```python
from build123d import *

# Parameters (mm, degrees)
EXTRUDE_1_DEPTH     = 12
SKETCH_2_R          = 3
SKETCH_2_R_2        = 0.81
CUT_EXTRUDE_1_DEPTH = 12
CUT_EXTRUDE_2_DEPTH = 8
FILLET_1_R          = 3
SKETCH_4_R          = 2.25
CUT_EXTRUDE_3_DEPTH = 10
CHAMFER_3_SIZE      = 3


with BuildPart() as part:
    # 草图1 → 凸台-拉伸1 (new body)
    with BuildSketch(Plane(origin=(0, 0, 0), x_dir=(1, 0, 0), z_dir=(0, 1, 0))):
        with BuildLine():
            Line((0, 0), (28, 0))
            ThreePointArc((28, 0), (30.121320344, 0.878679656), (31, 3))
            Line((31, 3), (31, 77))
            Line((31, 77), (-3, 77))
            Line((-3, 77), (-3, 3))
            ThreePointArc((-3, 3), (-2.121320344, 0.878679656), (0, 0))
        make_face()
    extrude(amount=EXTRUDE_1_DEPTH)

    # 草图2 → 切除-拉伸1 (cut)
    with BuildSketch(Plane(origin=(14.000000253, 12, -382.2), x_dir=(1, 0, 0), z_dir=(0, 1, 0))):
        with Locations(Location((13, -352.069110398, 0), (0, 0, 270))):
            Circle(SKETCH_2_R)
        with Locations(Location((-13, -352.069110398, 0), (0, 0, 270))):
            Circle(SKETCH_2_R)
        with Locations(Location((13, -378.069110398, 0), (0, 0, 270))):
            Circle(SKETCH_2_R)
        with Locations(Location((-13, -378.069110398, 0), (0, 0, 270))):
            Circle(SKETCH_2_R)
        with Locations(Location((-15.000000143, -309.999984702, 0), (0, 0, 270))):
            Circle(SKETCH_2_R_2)
        with Locations(Location((15.000000143, -309.999984702, 0), (0, 0, 270))):
            Circle(SKETCH_2_R_2)
        with Locations(Location((14.500000253, -365.000006616, 0), (0, 0, 270))):
            Circle(SKETCH_2_R_2)
        with Locations(Location((-14.500000253, -365.000006616, 0), (0, 0, 270))):
            Circle(SKETCH_2_R_2)
    extrude(amount=-CUT_EXTRUDE_1_DEPTH, mode=Mode.SUBTRACT)

    # 草图3 → 切除-拉伸2 (cut)
    with BuildSketch(Plane(origin=(14.000000253, 12, -382.2), x_dir=(1, 0, 0), z_dir=(0, 1, 0))):
        with BuildLine():
            Line((-7.000000134, -341.834781862), (-7.000000134, -355.639881164))
            ThreePointArc((-7.000000134, -355.639881164), (-7.313370109, -357.994123887), (-8.231657645, -360.184422392))
            ThreePointArc((-8.231657645, -360.184422392), (0, -374.536779603), (8.231657645, -360.184422392))
            ThreePointArc((8.231657645, -360.184422392), (7.313370109, -357.994123887), (7.000000134, -355.639881164))
            Line((7.000000134, -355.639881164), (7.000000134, -341.834782031))
            ThreePointArc((7.000000134, -341.834782031), (3.09e-07, -316.249981647), (-7.000000134, -341.834781862))
        make_face()
    extrude(amount=-CUT_EXTRUDE_2_DEPTH, mode=Mode.SUBTRACT)

    # 圆角1
    fillet_1_edges = [part.edges().sort_by_distance(p)[0] for p in [
        (-3, 6, -77),
        (31, 6, -77),
    ]]
    fillet(fillet_1_edges, radius=FILLET_1_R)

    # 草图4 → 切除-拉伸3 (cut)
    with BuildSketch(Plane.XZ):
        with Locations(Location((-0.5, -17.199993384, 0), (0, 0, 270))):
            Circle(SKETCH_4_R)
        with Locations(Location((28.500000507, -17.199993384, 0), (0, 0, 270))):
            Circle(SKETCH_4_R)
        with Locations((-0.99999989, -72.200015298)):
            Circle(SKETCH_4_R)
        with Locations((29.000000396, -72.200015298)):
            Circle(SKETCH_4_R)
    extrude(amount=-CUT_EXTRUDE_3_DEPTH, mode=Mode.SUBTRACT)

    # 倒角3
    # the kernel refuses this chamfer: 3 mm, written as the material it takes off along each edge
    with BuildSketch(Plane(origin=(0, 0, -74), x_dir=(-1, 0, 0), z_dir=(0, 0, 1))) as chamfer_3_piece_1:
        with BuildLine():
            Line((3 - CHAMFER_3_SIZE, 0), (3.084852814, -3.084852814))
            Line((3.084852814, -3.084852814), (3.144852814, -3.084852814))
            ThreePointArc((3.144852814, -3.084852814), (3.06, -1.542426407), (3.06, 0))
            Line((3.06, 0), (3, 0.06))
            Line((3, 0.06), (0, 0.142518829))
            Line((0, 0.142518829), (3 - CHAMFER_3_SIZE, 0))
        make_face()
    revolve(axis=Axis((0, 0, -74), (0, -1, 0)), revolution_arc=90, mode=Mode.SUBTRACT)
    with BuildSketch(Plane(origin=(-3, 0, -74), x_dir=(1, 0, 0), z_dir=(0, 0, 1))) as chamfer_3_piece_2:
        with BuildLine():
            Line((3.084852814, -0.084852814), (-0.084852814, 3.084852814))
            Line((-0.084852814, 3.084852814), (-0.144852814, 3.084852814))
            ThreePointArc((-0.144852814, 3.084852814), (-0.06, 1.542426407), (-0.06, 0))
            Line((-0.06, 0), (0, -0.06))
            ThreePointArc((0, -0.06), (1.542426407, -0.06), (3.084852814, -0.144852814))
            Line((3.084852814, -0.144852814), (3.084852814, -0.084852814))
        make_face()
    extrude(amount=8.484257474, mode=Mode.SUBTRACT)
    with BuildSketch(Plane(origin=(31, 0, -65.515743509), x_dir=(-1, 0, 0), z_dir=(0, 0, -1))) as chamfer_3_piece_3:
        with BuildLine():
            Line((3.084852814, -0.084852814), (-0.084852814, 3.084852814))
            Line((-0.084852814, 3.084852814), (-0.144852814, 3.084852814))
            ThreePointArc((-0.144852814, 3.084852814), (-0.06, 1.542426407), (-0.06, 0))
            Line((-0.06, 0), (0, -0.06))
            ThreePointArc((0, -0.06), (1.542426407, -0.06), (3.084852814, -0.144852814))
            Line((3.084852814, -0.144852814), (3.084852814, -0.084852814))
        make_face()
    extrude(amount=8.484256491, mode=Mode.SUBTRACT)
    with BuildSketch(Plane(origin=(28, 0, -74), x_dir=(1, 0, 0), z_dir=(0, 0, 1))) as chamfer_3_piece_4:
        with BuildLine():
            Line((3 - CHAMFER_3_SIZE, 0), (3.084852814, 3.084852814))
            Line((3.084852814, 3.084852814), (3.144852814, 3.084852814))
            ThreePointArc((3.144852814, 3.084852814), (3.06, 1.542426407), (3.06, 0))
            Line((3.06, 0), (3, -0.06))
            Line((3, -0.06), (0, -0.142518829))
            Line((0, -0.142518829), (3 - CHAMFER_3_SIZE, 0))
        make_face()
    revolve(axis=Axis((28, 0, -74), (0, 1, 0)), revolution_arc=90, mode=Mode.SUBTRACT)
    with BuildSketch(Plane(origin=(28, 0, -77), x_dir=(0, 0, 1), z_dir=(-1, 0, 0))) as chamfer_3_piece_5:
        with BuildLine():
            Line((3.084852814, -0.084852814), (-0.084852814, 3.084852814))
            Line((-0.084852814, 3.084852814), (-0.144852814, 3.084852814))
            ThreePointArc((-0.144852814, 3.084852814), (-0.06, 1.542426407), (-0.06, 0))
            Line((-0.06, 0), (0, -0.06))
            ThreePointArc((0, -0.06), (1.542426407, -0.06), (3.084852814, -0.144852814))
            Line((3.084852814, -0.144852814), (3.084852814, -0.084852814))
        make_face()
    extrude(amount=28, mode=Mode.SUBTRACT)
    # the kernel refuses this chamfer: 3 mm, written as the material it takes off along each edge
    with BuildSketch(Plane(origin=(-3, 0, -73.23079149), x_dir=(0, 1, 0), z_dir=(0, 0, 1))) as chamfer_3_2_piece_1:
        with BuildLine():
            Line((3.084852814, 0.084852814), (-0.084852814, -3.084852814))
            Line((-0.084852814, -3.084852814), (-0.144852814, -3.084852814))
            ThreePointArc((-0.144852814, -3.084852814), (-0.06, -1.542426407), (-0.06, 0))
            Line((-0.06, 0), (0, 0.06))
            ThreePointArc((0, 0.06), (1.542426407, 0.06), (3.084852814, 0.144852814))
            Line((3.084852814, 0.144852814), (3.084852814, 0.084852814))
        make_face()
    extrude(amount=70.23079149, mode=Mode.SUBTRACT)
    with BuildSketch(Plane(origin=(0, 0, -3), x_dir=(-1, 0, 0), z_dir=(0, 0, -1))) as chamfer_3_2_piece_2:
        with BuildLine():
            Line((3 - CHAMFER_3_SIZE, 0), (3.084852814, 3.084852814))
            Line((3.084852814, 3.084852814), (3.144852814, 3.084852814))
            ThreePointArc((3.144852814, 3.084852814), (3.06, 1.542426407), (3.06, 0))
            Line((3.06, 0), (3, -0.06))
            Line((3, -0.06), (0, -0.142518829))
            Line((0, -0.142518829), (3 - CHAMFER_3_SIZE, 0))
        make_face()
    revolve(axis=Axis((0, 0, -3), (0, 1, 0)), revolution_arc=90, mode=Mode.SUBTRACT)
    with BuildSketch(Plane(origin=(0, 0, 0), x_dir=(0, 0, -1), z_dir=(1, 0, 0))) as chamfer_3_2_piece_3:
        with BuildLine():
            Line((3.084852814, -0.084852814), (-0.084852814, 3.084852814))
            Line((-0.084852814, 3.084852814), (-0.144852814, 3.084852814))
            ThreePointArc((-0.144852814, 3.084852814), (-0.06, 1.542426407), (-0.06, 0))
            Line((-0.06, 0), (0, -0.06))
            ThreePointArc((0, -0.06), (1.542426407, -0.06), (3.084852814, -0.144852814))
            Line((3.084852814, -0.144852814), (3.084852814, -0.084852814))
        make_face()
    extrude(amount=28, mode=Mode.SUBTRACT)
    with BuildSketch(Plane(origin=(28, 0, -3), x_dir=(0, 0, 1), z_dir=(-1, 0, 0))) as chamfer_3_2_piece_4:
        with BuildLine():
            Line((3 - CHAMFER_3_SIZE, 0), (3.084852814, 3.084852814))
            Line((3.084852814, 3.084852814), (3.144852814, 3.084852814))
            ThreePointArc((3.144852814, 3.084852814), (3.06, 1.542426407), (3.06, 0))
            Line((3.06, 0), (3, -0.06))
            Line((3, -0.06), (0, -0.142518829))
            Line((0, -0.142518829), (3 - CHAMFER_3_SIZE, 0))
        make_face()
    revolve(axis=Axis((28, 0, -3), (0, 1, 0)), revolution_arc=90, mode=Mode.SUBTRACT)
    with BuildSketch(Plane(origin=(31, 0, -3), x_dir=(-1, 0, 0), z_dir=(0, 0, -1))) as chamfer_3_2_piece_5:
        with BuildLine():
            Line((3.084852814, -0.084852814), (-0.084852814, 3.084852814))
            Line((-0.084852814, 3.084852814), (-0.144852814, 3.084852814))
            ThreePointArc((-0.144852814, 3.084852814), (-0.06, 1.542426407), (-0.06, 0))
            Line((-0.06, 0), (0, -0.06))
            ThreePointArc((0, -0.06), (1.542426407, -0.06), (3.084852814, -0.144852814))
            Line((3.084852814, -0.144852814), (3.084852814, -0.084852814))
        make_face()
    extrude(amount=70.230792473, mode=Mode.SUBTRACT)


solid = part.part
```
Could you check a few things on this model? Use its own coordinates, in mm. A direction names the side the tool comes from. Round coordinates to 2 decimals unless told otherwise and drop trailing zeros. Loops run counter-clockwise (first coordinate to the right, second up) from the corner with the lowest first, then second, coordinate; pieces in that order, holes last.
Q1. For P1, Ø14, axis at x = 11, z = -51, coming from the +Y side; P2, Ø2, axis at x = -0.5, z = -17.2, coming from the -Y side; P3, Ø5.5, axis at x = 1, z = -30.13, coming from the -Y side, each with a flat end and sliding along its axis, tell me the tip position at first contact or that it passes through.
Q2. I want a section at B-B (x = 14). Write out the boundary of the cut face in (y, z), and give its area (3 significant figures).
Q3. On a 3-axis mill with a long thin cutter (end or side, diameter ignored), from which of +Z, -Z, +X, -X, +Y, -Y can I reach the whole of each face in a straight line? I mean faces 1 (the cylindrical face through (-2.14, 7.44, -0.9)), 2 (the flat face through (27.5, 10, -17.2)), 3 (the cylindrical face through (6.695, 8.056, -24.238)). Say none if no direction works.
Q4. Thinking about a two-plate mould opening in Z: for faces 4 (the flat face through (21, 8, -33)), 5 (the conical face through (29.577, 2.256, -1.388)), 6 (the conical face through (-1.163, 1.627, -75.138)), which applies, pulls with the +Z half, pulls with the -Z half, needs draft (parallel to the pull), parting line crosses it, or undercut?
Q5. Please list where these lines run through material, in increasing order: L1, parallel to Z at x = 29, y = 7.25; L2, parallel to Z at x = 13.5, y = 7.25; L3, parallel to X at y = 11.25, z = -31.
Q6. I want a section at D-D (z = -67). Write out the boundary of the cut face in (x, y), and give its area (3 significant figures).
Q7. I want a section at C-C (z = -34). Write out the boundary of the cut face in (x, y).
Q8. I want a section at A-A (y = 8.5). Write out the boundary of the cut face in (x, z), and give its area (3 significant figures).
Answer below:
1. P1: stops at y = 4
1. P2: stops at y = 10
1. P3: passes through
2. outline: (0, -74) - (3, -77) - (12, -77) - (12, -65.95) - (4, -65.95) - (4, -7.66) - (12, -7.66) - (12, 0) - (3, 0) - (0, -3) - close
2. area: 449 mm2
3. face 1: +Z, -X, +Y, -Y
3. face 2: -Y
3. face 3: +Y
4. face 4: undercut
4. face 5: pulls with the +Z half
4. face 6: pulls with the -Z half
5. L1: z = -76.83 to -74.45, -69.95 to -32.37, -27.89 to -19.39, -15.01 to -6.37, -1.89 to -0.17
5. L2: z = -77 to -65.94, -7.68 to 0
5. L3: x = -3 to -1.87, 3.87 to 7, 21 to 24.13, 29.87 to 31
6. outline: (-3, 3) - (0, 0) - (28, 0) - (31, 3) - (31, 12) - (-3, 12) - close
6. area: 399 mm2
7. outline: (-3, 3) - (0, 0) - (28, 0) - (31, 3) - (31, 12) - (21, 12) - (21, 4) - (7, 4) - (7, 12) - (-3, 12) - close
8. outline: (-3, -74) arc R3 ccw to (0, -77) - (28, -77) arc R3 ccw to (31, -74) - (31, -73.23) arc R2.25 cw (long way) to (31, -71.17) - (31, -3) arc R3 ccw to (28, 0) - (0, 0) arc R3 ccw to (-3, -3) - (-3, -71.17) arc R2.25 cw (long way) to (-3, -73.23) - close; hole circle Ø4.5 at (-0.5, -17.2); hole circle Ø6 at (1, -30.13); hole circle Ø6 at (1, -4.13); hole (5.77, -22.02) arc R9 cw to (7, -26.56) - (7, -40.37) arc R13.75 ccw (long way) to (21, -40.37) - (21, -26.56) arc R9 cw to (22.23, -22.02) arc R9.54 ccw (long way) to start; hole circle Ø6 at (27, -30.13); hole circle Ø6 at (27, -4.13); hole circle Ø4.5 at (28.5, -17.2)
8. area: 1,370 mm2
